Geometry: final body of the model. Coordinates: model frame, mm. Round coordinates to 2 decimals unless told otherwise and drop trailing zeros. Order: outer loops, then holes, each group sorted by start corner. A loop starts at its lowest first (then second) coordinate and runs counter-clockwise, first axis right, second up. Notation, with made-up numbers: M 58,86.5 L 106,86.5 A31 cw 106,114.5 Z; hole C -2.5,81 d5. An arc over 180 degrees is marked long. Return JSON: item names as keys, results as strings. Group by question number.
Q1. Mould query, pull axis Z, two halves, no side actions, for faces 1 (the face through (0, 65, 2)), 2 (the face through (0.748, -0.907, -0.976)), 3 (the face through (-3, -0.9, 1.8)). Classes: released by +Z, released by -Z, zero draft, split by the parting line, or undercut.
Q2. Contact query for a flat-ended pin moving along its axis: pin 1 (1 mm diameter, centred on y = -22, z = -2, fed in from -X). Output: stop coordinate, or through.
Q3. Cut plane B-B on y = -22.5. Output: boundary loops of the cut face in (x, z), and give its area (3 significant figures).
Q4. Ray query, probe 1 along X at (y, z) = (3.5, 0); probe 2 along Z at (x, y) = (0, 38); probe 3 along Z at (x, y) = (0.5, -37.5). Return the intervals inside material, ascending.
Q5. Cut plane A-A on x = 0. Output: boundary loops of the cut face in (y, z), and give its area (3 significant figures).
Autodesk Inventor part; units mm, degrees
ref_plane "YZ Plane" through (0, 0, 0) normal (1, 0, 0) x (0, 1, 0)
ref_plane "XZ Plane" through (0, 0, 0) normal (0, 1, 0) x (-1, 0, 0)
ref_plane "XY Plane" through (0, 0, 0) normal (0, 0, 1) x (1, 0, 0)
sketch "スケッチ1" plane through (0, 0, 0) normal (0, 1, 0) x (-1, 0, 0)
  line L0 (2.0207, 3.5) -> (4.0415, 0)
  line L1 (4.0415, 0) -> (2.0207, -3.5)
  line L2 (2.0207, -3.5) -> (-2.0207, -3.5)
  line L3 (-2.0207, -3.5) -> (-4.0415, 0)
  line L4 (-4.0415, 0) -> (-2.0207, 3.5)
  line L5 (-2.0207, 3.5) -> (2.0207, 3.5)
  point P0 (0, 0)
  point P1 (0, 0)
  dimension "d0" = 7
extrude "押し出し1" add sketch "スケッチ1" along normal mid plane 130
sketch "スケッチ2" plane through (0, 65, 0) normal (0, 1, 0) x (1, 0, 0)
  point P0 (0, 0)
  point P1 (0, 0)
hole "穴1" at (0, 65, 0) direction (0, -1, 0) diameter 2.459 end through all
chamfer "面取り1" distance 0.2 angle 45 2 edges at (0, 65, -1.2295) (0, -65, -1.2295)
chamfer "面取り2" distance 0.2 angle 45 12 edges at (0, 65, 3.5) (-3.0311, 65, 1.75) (-3.0311, 65, -1.75) (0, 65, -3.5) (3.0311, 65, -1.75) (3.0311, 65, 1.75) (3.0311, -65, 1.75) (3.0311, -65, -1.75) (0, -65, 3.5) (-3.0311, -65, 1.75) (-3.0311, -65, -1.75) (0, -65, -3.5)
properties part number "Spacer_M3-Hex7-L130"
Result sheet:
{
 "1": {"face 1": "zero draft", "face 2": "undercut", "face 3": "released by +Z"},
 "2": {"pin 1": "stops at x = -3.18"},
 "3": {"outline": "M -4.04,0 L -2.02,-3.5 L 2.02,-3.5 L 4.04,0 L 2.02,3.5 L -2.02,3.5 Z; hole C 0,0 d2.46", "area": "37.7 mm²"},
 "4": {"probe 1": "x = -4.04 to -1.23, 1.23 to 4.04", "probe 2": "z = -3.5 to -1.23, 1.23 to 3.5", "probe 3": "z = -3.5 to -1.12, 1.12 to 3.5"},
 "5": {"outline": "M -65,-3.3 L -64.8,-3.5 L 64.8,-3.5 L 65,-3.3 L 65,-1.43 L 64.8,-1.23 L -64.8,-1.23 L -65,-1.43 Z; M -65,1.43 L -64.8,1.23 L 64.8,1.23 L 65,1.43 L 65,3.3 L 64.8,3.5 L -64.8,3.5 L -65,3.3 Z", "area": "590 mm²"}
}
